Design review of the part built by this model. Coordinates are the model's own, in mm. A direction names the side the tool comes from. Round coordinates to 2 decimals unless told otherwise and drop trailing zeros. Write each loop counter-clockwise with the first axis right and the second up, starting at its lowest first coordinate (ties: lowest second). Pieces come first, ordered by that corner, then holes. Notation, with made-up numbers: (-26.75, 15) -> (13.25, 15) arc R21 ccw to (13.25, 37) -> close; hole circle Ø5 at (70, 46.25). An arc over 180 degrees is marked (long way). Write item = value, one per line. Start each with the question number.
Item 1: To check wall thickness, follow L1, parallel to X at y = 0.25, z = 4; L2, parallel to Y at x = -48, z = 9; L3, parallel to Y at x = -53, z = 7.5. State the ranges of each line that lie inside material, in increasing order.
Item 2: Add section D-D, the plane z = 6. State the section outline as (x, y) points.
Item 3: Add section C-C, the plane x = -64. State the section outline as (y, z) points.
Item 4: Mouldability with a two-part tool opening along Y and no side actions: class faces 1 (the cylindrical face through (-35.78, 19.25, 1.48)), 2 (the flat face through (-56, 19, 3)), 3 (the cylindrical face through (-70.5, -1.776, 1.479)), 4 (the flat face through (-49, -3.318, 14)) as released by +Y, released by -Y, zero draft, split by the parting line, or undercut.
Item 5: Add section B-B, the plane y = 9.5. State the section outline as (x, z) points, then the cut area to 3 significant figures.
Item 6: Machinability: for faces 5 (the flat face through (-55, 14.96, 12)), 6 (the flat face through (-57, -7.04, 1)), 7 (the flat face through (-45.407, 4, 7)), which of the approach directions +Z, -Z, +X, -X, +Y, -Y give a long, thin tool a straight path to every point of the face, cutting with its end or side? Answer none if there is none.
Item 7: Add section A-A, the plane z = 12. State the section outline as (x, y) points, then the cut area to 3 significant figures.
Item 8: For pin 1 Ø1.5 at (x, z) = (-61.5, 5) entering from -Y; pin 2 Ø2.5 at (y, z) = (4, 6) entering from -X; pin 3 Ø1.6 at (x, z) = (-46, 12.5) entering from +Y, all flat-tipped, find the tip position at first contact; note any pin that passes through.
from build123d import *

# Parameters (mm, degrees)
CROQUIS1_R              = 1.5
SALIENTE_EXTRUIR1_DEPTH = 3
SALIENTE_EXTRUIR2_DEPTH = 8
CROQUIS3_W              = 13
CROQUIS3_H              = 1.7
CORTAR_EXTRUIR1_DEPTH   = 8
CROQUIS5_W              = 3.5
CROQUIS5_H              = 11
CROQUIS5_W_2            = 6.5
SALIENTE_EXTRUIR3_DEPTH = 1.5
SALIENTE_EXTRUIR4_DEPTH = 4
CORTAR_EXTRUIR2_START   = -22.8
CROQUIS11_W             = 2
CROQUIS11_H             = 20
CORTAR_EXTRUIR2_DEPTH   = 22.8


with BuildPart() as part:
    # Croquis1 → Saliente-Extruir1 (new body)
    with BuildSketch(Plane.XY):
        with BuildLine():
            Line((-75.306602598, 17.959617496), (-75.306602598, -7.040382504))
            Line((-75.306602598, -7.040382504), (-35.306602598, -7.040382504))
            Line((-35.306602598, -7.040382504), (-35.306602598, 17.959617496))
            ThreePointArc((-35.306602598, 17.959617496), (-35.791122177, 19.26473017), (-37.009921692, 19.937490201))
            Line((-37.009921692, 19.937490201), (-73.603283504, 19.937490201))
            ThreePointArc((-73.603283504, 19.937490201), (-74.822083019, 19.26473017), (-75.306602598, 17.959617496))
        make_face()
        with Locations((-71.306602598, -3.040382504)):
            Circle(CROQUIS1_R, mode=Mode.SUBTRACT)
        with Locations((-39.306602598, -3.040382504)):
            Circle(CROQUIS1_R, mode=Mode.SUBTRACT)
    extrude(amount=SALIENTE_EXTRUIR1_DEPTH)

    # Croquis2 → Saliente-Extruir2 (add)
    with BuildSketch(Plane.XY.offset(3)):
        Polygon((-66.706602598, -7.040382504), (-65.206602598, -7.040382504), (-65.206602598, 14.959617496), (-45.406602598, 14.959617496), (-45.406602598, -7.040382504), (-43.906602598, -7.040382504), (-43.906602598, 16.459617496), (-66.706602598, 16.459617496), align=None)
    extrude(amount=SALIENTE_EXTRUIR2_DEPTH)

    # Croquis3 → Cortar-Extruir1 (cut)
    with BuildSketch(Plane.XZ.offset(7.040382504)):
        with Locations((-58.706602598, 2.15)):
            Rectangle(CROQUIS3_W, CROQUIS3_H)
    extrude(amount=-CORTAR_EXTRUIR1_DEPTH, mode=Mode.SUBTRACT)

    # Croquis5 → Saliente-Extruir3 (add)
    with BuildSketch(Plane.XZ.offset(7.040382504)):
        with Locations((-64.956602598, 5.5)):
            Rectangle(CROQUIS5_W, CROQUIS5_H)
        with Locations((-47.156602598, 5.5)):
            Rectangle(CROQUIS5_W_2, CROQUIS5_H)
    extrude(amount=SALIENTE_EXTRUIR3_DEPTH)

    # Croquis6 → Saliente-Extruir4 (add)
    with BuildSketch(Plane.XY.offset(11)):
        Polygon((-63.206602598, -7.040382504), (-63.206602598, -8.540382504), (-66.706602598, -8.540382504), (-66.706602598, 16.459617496), (-43.906602598, 16.459617496), (-43.906602598, -8.540382504), (-50.406602598, -8.540382504), (-50.406602598, -3.318007663), (-47.406602598, -3.318007663), (-47.406602598, 14.681992337), (-63.206602598, 14.681992337), align=None)
    extrude(amount=SALIENTE_EXTRUIR4_DEPTH)

    # Croquis11 → Cortar-Extruir2 (cut)
    with BuildSketch(Plane.ZY.offset(66.706602598).offset(CORTAR_EXTRUIR2_START)):
        with Locations((12.5, 4.959617496)):
            Rectangle(CROQUIS11_W, CROQUIS11_H)
    extrude(amount=CORTAR_EXTRUIR2_DEPTH, mode=Mode.SUBTRACT)


solid = part.part
Result set:
q1.L1 = -66.71 to -65.21, -45.41 to -43.91
q1.L2 = -8.54 to -7.04, 14.96 to 16.46
q1.L3 = 14.96 to 16.46
q2.outline = (-66.71, -8.54) -> (-63.21, -8.54) -> (-63.21, -7.04) -> (-65.21, -7.04) -> (-65.21, 14.96) -> (-45.41, 14.96) -> (-45.41, -7.04) -> (-50.41, -7.04) -> (-50.41, -8.54) -> (-43.91, -8.54) -> (-43.91, 16.46) -> (-66.71, 16.46) -> close
q3.outline = (-8.54, 0) -> (19.94, 0) -> (19.94, 3) -> (16.46, 3) -> (16.46, 15) -> (-8.54, 15) -> close; hole (-7.04, 1.3) -> (0.96, 1.3) -> (0.96, 3) -> (14.96, 3) -> (14.96, 11) -> (-7.04, 11) -> close; hole (-5.04, 11.5) -> (14.96, 11.5) -> (14.96, 13.5) -> (-5.04, 13.5) -> close
q4.face_1 = released by +Y
q4.face_2 = zero draft
q4.face_3 = undercut
q4.face_4 = undercut
q5.outline = (-75.31, 0) -> (-35.31, 0) -> (-35.31, 3) -> (-43.91, 3) -> (-43.91, 11.5) -> (-47.41, 11.5) -> (-47.41, 11) -> (-45.41, 11) -> (-45.41, 3) -> (-65.21, 3) -> (-65.21, 11) -> (-63.21, 11) -> (-63.21, 11.5) -> (-66.71, 11.5) -> (-66.71, 3) -> (-75.31, 3) -> close; (-66.71, 13.5) -> (-63.21, 13.5) -> (-63.21, 15) -> (-66.71, 15) -> close; (-47.41, 13.5) -> (-43.91, 13.5) -> (-43.91, 15) -> (-47.41, 15) -> close
q5.area = 158 mm²
q6.face_5 = +X, -X
q6.face_6 = +Z, -Z, -Y
q6.face_7 = none
q7.outline = (-66.71, -8.54) -> (-63.21, -8.54) -> (-63.21, -5.04) -> (-66.71, -5.04) -> close; (-66.71, 14.96) -> (-43.91, 14.96) -> (-43.91, 16.46) -> (-66.71, 16.46) -> close; (-50.41, -8.54) -> (-43.91, -8.54) -> (-43.91, -5.04) -> (-50.41, -5.04) -> close
q7.area = 69.2 mm²
q8.pin_1 = 14.96
q8.pin_2 = -66.71
q8.pin_3 = 16.46
